Input: part model. Units: mm. Frame: model coordinates. A direction names the side the tool comes from. Coordinates: 2 decimals unless noted, no trailing zeros. Write each loop counter-clockwise with the first axis right and the second up, starting at its lowest first coordinate (ties: lowest second). Pieces come first, ordered by that corner, then holes.
1) Pin query (flat end, axial travel): pin 1 Ø3 at (x, z) = (0, 10) entering from +Y (3 decimals); pin 2 Ø3 at (x, z) = (-1, -30) entering from +Y; pin 3 Ø4 at (x, z) = (0, -10) entering from -Y. Return the tip coordinate at first contact, or that it passes through.
2) Section query B-B (z = 22). Output: boundary loops of the cut face in (x, y).
3) Set-up query: faces 4 (the flat face through (0, -0.25, -12)), 5 (the cylindrical face through (0.39, -1.581, 8.243)). Return all of +Z, -Z, +X, -X, +Y, -Y with unobstructed straight access to the full face (end or side cutting, diameter ignored); none if empty.
4) Draft query along Z for faces 1 (the flat face through (-4.5, -1, -1)), 2 (the flat face through (0, 0, 37.5)), 3 (the cylindrical face through (0.234, -1.581, 31.785)). Return one class per face: pulls with the +Z half, pulls with the -Z half, needs draft (parallel to the pull), parting line crosses it, or undercut.
5) Section query C-C (x = 0). State how many separate pieces and enclosed holes the cut face has, then the cut area to 3 significant figures.
6) Line query: L1, parallel to Z at x = 0, y = 1.4; L2, parallel to Z at x = 0, y = -2; L3, parallel to Y at x = -3.75, z = 17.5. Output: solid intervals per line, ascending.
Autodesk Inventor part; units mm, degrees
ref_plane "to_block1_XY" through (0, -3.25, 0) normal (0, 0, 1) x (1, 0, 0)
ref_plane "to_block1_YZ" through (0, -3.25, 0) normal (1, 0, 0) x (0, 1, 0)
ref_plane "to_block1_ZX" through (0, -3.25, 0) normal (0, 1, 0) x (0, 0, 1)
sketch "_____1" plane through (0, 0, 0) normal (0, 0, 1) x (1, 0, 0)
  line L0 (-4.5, 2.95) -> (-4.5, 2.1665)
  arc A0 (-3.9835, 1.65) -> (-4.5, 2.1665) centre (-4.9, 1.25) ccw
  line L1 (-3.9835, 1.65) -> (-3.6, 1.65)
  arc A1 (-3.6, 0.85) -> (-3.6, 1.65) centre (-3.6, 1.25) ccw
  line L2 (-3.6, 0.85) -> (-3.9835, 0.85)
  arc A2 (-4.5, 0.3335) -> (-3.9835, 0.85) centre (-4.9, 1.25) ccw
  line L3 (-4.5, 0.3335) -> (-4.5, -2.95)
  line L4 (-4.5, -2.95) -> (-4.2, -3.25)
  line L5 (-4.2, -3.25) -> (4.2, -3.25)
  line L6 (4.2, -3.25) -> (4.5, -2.95)
  line L7 (4.5, -2.95) -> (4.5, 0.3335)
  arc A3 (3.9835, 0.85) -> (4.5, 0.3335) centre (4.9, 1.25) ccw
  line L8 (3.9835, 0.85) -> (3.6, 0.85)
  arc A4 (3.6, 1.65) -> (3.6, 0.85) centre (3.6, 1.25) ccw
  line L9 (3.6, 1.65) -> (3.9835, 1.65)
  arc A5 (4.5, 2.1665) -> (3.9835, 1.65) centre (4.9, 1.25) ccw
  line L10 (4.5, 2.1665) -> (4.5, 2.95)
  line L11 (4.5, 2.95) -> (4.2, 3.25)
  line L12 (4.2, 3.25) -> (-4.2, 3.25)
  line L13 (-4.2, 3.25) -> (-4.5, 2.95)
extrude "Extrusion1" add sketch "_____1" along normal mid plane 75
sketch "_____5" plane through (0, 0, 30) normal (0, 0, 1) x (1, 0, 0)
  line L0 (0, 3.25) -> (0, -3.25)
  line L1 (0, -3.25) -> (-2.1, -3.25)
  line L2 (-2.1, -3.25) -> (-1.8, -2.95)
  line L3 (-1.8, -2.95) -> (-1.8, -0.25)
  line L4 (-1.8, -0.25) -> (-3, -0.25)
  line L5 (-3, -0.25) -> (-3, 2.95)
  line L6 (-3, 2.95) -> (-3.3, 3.25)
  line L7 (-3.3, 3.25) -> (0, 3.25)
  line L8 (0, 3.25) -> (0, -3.25)
revolve "Revolution1" cut sketch "_____5" angle 360 about axis through (0, 3.25, 30) along (0, 1, 0)
pattern_linear "Rectangular Pattern1" count 4 spacing 20 along (0, 0, -1) of "Revolution1"
ref_plane "to_block1_XY" through (0, -3.25, 0) normal (0, 0, 1) x (1, 0, 0)
ref_plane "to_block1_YZ" through (0, -3.25, 0) normal (1, 0, 0) x (0, 1, 0)
ref_plane "to_block1_ZX" through (0, -3.25, 0) normal (0, 1, 0) x (0, 0, 1)
properties part number "C-MLG9-75_r"
Answer:
1. pin 1: passes through
1. pin 2: stops at y = -0.25
1. pin 3: stops at y = -3.15
2. outline: (-4.5, -2.95) - (-4.2, -3.25) - (4.2, -3.25) - (4.5, -2.95) - (4.5, 0.33) arc R1 cw to (3.98, 0.85) - (3.6, 0.85) arc R0.4 cw to (3.6, 1.65) - (3.98, 1.65) arc R1 cw to (4.5, 2.17) - (4.5, 2.95) - (4.2, 3.25) - (-4.2, 3.25) - (-4.5, 2.95) - (-4.5, 2.17) arc R1 cw to (-3.98, 1.65) - (-3.6, 1.65) arc R0.4 cw to (-3.6, 0.85) - (-3.98, 0.85) arc R1 cw to (-4.5, 0.33) - close
3. face 4: +Y
3. face 5: +Y, -Y
4. face 1: needs draft
4. face 2: pulls with the +Z half
4. face 3: undercut
5. separate pieces: 5
5. enclosed holes: 0
5. area: 360 mm2
6. L1: z = -37.5 to -33, -27 to -13, -7 to 7, 13 to 27, 33 to 37.5
6. L2: z = -37.5 to -31.8, -28.2 to -11.8, -8.2 to 8.2, 11.8 to 28.2, 31.8 to 37.5
6. L3: y = -3.25 to 0.85, 1.65 to 3.25
